from build123d import *

# Parameters (mm, degrees)
SKETCH1_R                          = 5.1
BOSS_EXTRUDE1_DEPTH                = 70.75
FURO_ROSCADO_DE_M5X0_81_AT_2_COUNT = 2
FURO_ROSCADO_DE_M5X0_81_AT_2_PITCH = 32
M3X0_5_TAPPED_HOLE1_AT_2_COUNT     = 2
M3X0_5_TAPPED_HOLE1_AT_2_PITCH     = 11.313708499
M3X0_5_TAPPED_HOLE1_AT_3_COUNT     = 2
M3X0_5_TAPPED_HOLE1_AT_3_PITCH     = 11.313708499
M3X0_5_TAPPED_HOLE1_AT_4_COUNT     = 2
M3X0_5_TAPPED_HOLE1_AT_4_PITCH     = 16
FURO_ROSCADO_DE_M4X0_71_AT_2_COUNT = 2
FURO_ROSCADO_DE_M4X0_71_AT_2_PITCH = 42
PADR_O_LINEAR1_COUNT               = 2
PADR_O_LINEAR1_PITCH               = 180
SKETCH5_W                          = 100
SKETCH5_H                          = 30
BOSS_EXTRUDE2_DEPTH                = 141.5
LPATTERN1_COUNT                    = 2
LPATTERN1_PITCH                    = 140


with BuildPart() as part:
    # Sketch1 → Boss-Extrude1 (new, symmetric)
    with BuildSketch(Plane.XY):
        with BuildLine():
            Line((-140, 0), (-140, 26))
            Line((-140, 26), (140, 26))
            Line((140, 26), (140, 0))
            Line((140, 0), (101.674330816, 0))
            ThreePointArc((101.674330816, 0), (90, 7.7), (78.325669184, 0))
            Line((78.325669184, 0), (-78.325669184, 0))
            ThreePointArc((-78.325669184, 0), (-90, 7.7), (-101.674330816, 0))
            Line((-101.674330816, 0), (-140, 0))
        make_face()
        with Locations((0, 15)):
            Circle(SKETCH1_R, mode=Mode.SUBTRACT)
    extrude(amount=BOSS_EXTRUDE1_DEPTH, both=True)

    # Esboço3 → Furo roscado de M5x0.81 (revolve, cut)
    with BuildSketch(Plane(origin=(110, 26, -50), x_dir=(0, 0, 1), z_dir=(1, 0, 0))):
        Polygon((0, 0), (0, 15.2618073), (2.1, 14), (2.1, 0.425), (2.525, 0), align=None)
    furo_roscado_de_m5x0_81 = revolve(axis=Axis((110, 32.35, -50), (0, -1, 0)), mode=Mode.SUBTRACT)

    # Furo roscado de M5x0.81 at 2: Furo roscado de M5x0.81 ×2
    with Locations(*[(0, 0, i * FURO_ROSCADO_DE_M5X0_81_AT_2_PITCH) for i in range(1, FURO_ROSCADO_DE_M5X0_81_AT_2_COUNT)]):
        add(furo_roscado_de_m5x0_81, mode=Mode.SUBTRACT)

    # Sketch4 → M3x0.5 Tapped Hole1 (revolve, cut)
    with BuildSketch(Plane(origin=(-5.656854249, 20.656854249, 70.75), x_dir=(0, -1, 0), z_dir=(1, 0, 0))):
        Polygon((0, 0), (0, 13.251075774), (1.25, 12.5), (1.25, 0), align=None)
    m3x0_5_tapped_hole1 = revolve(axis=Axis((-5.656854249, 20.656854249, 77.1), (0, 0, -1)), mode=Mode.SUBTRACT)

    # M3x0.5 Tapped Hole1 at 2: M3x0.5 Tapped Hole1 ×2
    with Locations(*[(i * M3X0_5_TAPPED_HOLE1_AT_2_PITCH, 0, 0) for i in range(1, M3X0_5_TAPPED_HOLE1_AT_2_COUNT)]):
        add(m3x0_5_tapped_hole1, mode=Mode.SUBTRACT)

    # M3x0.5 Tapped Hole1 at 3: M3x0.5 Tapped Hole1 ×2
    with Locations(*[(0, -i * M3X0_5_TAPPED_HOLE1_AT_3_PITCH, 0) for i in range(1, M3X0_5_TAPPED_HOLE1_AT_3_COUNT)]):
        add(m3x0_5_tapped_hole1, mode=Mode.SUBTRACT)

    # M3x0.5 Tapped Hole1 at 4: M3x0.5 Tapped Hole1 ×2
    with Locations(*[Vector(0.7071067811865596, -0.7071067811865357, 0) * (i * M3X0_5_TAPPED_HOLE1_AT_4_PITCH) for i in range(1, M3X0_5_TAPPED_HOLE1_AT_4_COUNT)]):
        add(m3x0_5_tapped_hole1, mode=Mode.SUBTRACT)

    # Mirror2: M3x0.5 Tapped Hole1 across plane
    add(m3x0_5_tapped_hole1.mirror(Plane.XY), mode=Mode.SUBTRACT)

    # Mirror2 copy 1 sketch → Mirror2 copy 1 (revolve, cut)
    with BuildSketch(Plane(origin=(5.656854249, 20.656854249, -70.75), x_dir=(0, -1, 0), z_dir=(1, 0, 0))):
        Polygon((0, 0), (0, -13.251075774), (1.25, -12.5), (1.25, 0), align=None)
    revolve(axis=Axis((5.656854249, 20.656854249, -77.1), (0, 0, -1)), mode=Mode.SUBTRACT)

    # Mirror2 copy 2 sketch → Mirror2 copy 2 (revolve, cut)
    with BuildSketch(Plane(origin=(-5.656854249, 9.343145751, -70.75), x_dir=(0, -1, 0), z_dir=(1, 0, 0))):
        Polygon((0, 0), (0, -13.251075774), (1.25, -12.5), (1.25, 0), align=None)
    revolve(axis=Axis((-5.656854249, 9.343145751, -77.1), (0, 0, -1)), mode=Mode.SUBTRACT)

    # Mirror2 copy 3 sketch → Mirror2 copy 3 (revolve, cut)
    with BuildSketch(Plane(origin=(5.656854249, 9.343145751, -70.75), x_dir=(0, -1, 0), z_dir=(1, 0, 0))):
        Polygon((0, 0), (0, -13.251075774), (1.25, -12.5), (1.25, 0), align=None)
    revolve(axis=Axis((5.656854249, 9.343145751, -77.1), (0, 0, -1)), mode=Mode.SUBTRACT)

    # Esboço7 → Furo roscado de M4x0.71 (revolve, cut)
    with BuildSketch(Plane(origin=(-55, 26, -21), x_dir=(0, 0, 1), z_dir=(1, 0, 0))):
        Polygon((0, 0), (0, 12.491420021), (1.65, 11.5), (1.65, 0.375), (2.025, 0), align=None)
    furo_roscado_de_m4x0_71 = revolve(axis=Axis((-55, 32.35, -21), (0, -1, 0)), mode=Mode.SUBTRACT)

    # Furo roscado de M4x0.71 at 2: Furo roscado de M4x0.71 ×2
    with Locations(*[(0, 0, i * FURO_ROSCADO_DE_M4X0_71_AT_2_PITCH) for i in range(1, FURO_ROSCADO_DE_M4X0_71_AT_2_COUNT)]):
        add(furo_roscado_de_m4x0_71, mode=Mode.SUBTRACT)

    # Padrão linear1: Furo roscado de M4x0.71 ×2
    with Locations(*[(i * PADR_O_LINEAR1_PITCH, 0, 0) for i in range(1, PADR_O_LINEAR1_COUNT)]):
        add(furo_roscado_de_m4x0_71, mode=Mode.SUBTRACT)

    # Padrão linear1 copy 1 sketch → Padrão linear1 copy 1 (revolve, cut)
    with BuildSketch(Plane(origin=(125, 26, 21), x_dir=(0, 0, 1), z_dir=(1, 0, 0))):
        Polygon((0, 0), (0, 12.491420021), (1.65, 11.5), (1.65, 0.375), (2.025, 0), align=None)
    revolve(axis=Axis((125, 32.35, 21), (0, -1, 0)), mode=Mode.SUBTRACT)

    # Sketch5 → Boss-Extrude2 (add)
    with BuildSketch(Plane.XY.offset(70.75)):
        with Locations((0, -15)):
            Rectangle(SKETCH5_W, SKETCH5_H)
    extrude(amount=-BOSS_EXTRUDE2_DEPTH)

    # LPattern1: Furo roscado de M5x0.81 ×2
    with Locations(*[(-i * LPATTERN1_PITCH, 0, 0) for i in range(1, LPATTERN1_COUNT)]):
        add(furo_roscado_de_m5x0_81, mode=Mode.SUBTRACT)

    # LPattern1 copy 1 sketch → LPattern1 copy 1 (revolve, cut)
    with BuildSketch(Plane(origin=(-30, 26, -18), x_dir=(0, 0, 1), z_dir=(1, 0, 0))):
        Polygon((0, 0), (0, 15.2618073), (2.1, 14), (2.1, 0.425), (2.525, 0), align=None)
    revolve(axis=Axis((-30, 32.35, -18), (0, -1, 0)), mode=Mode.SUBTRACT)

    # Mirror3: Furo roscado de M5x0.81 across plane
    add(furo_roscado_de_m5x0_81.mirror(Plane.XY), mode=Mode.SUBTRACT)

    # Mirror3 copy 1 sketch → Mirror3 copy 1 (revolve, cut)
    with BuildSketch(Plane(origin=(110, 26, 18), x_dir=(0, 0, -1), z_dir=(1, 0, 0))):
        Polygon((0, 0), (0, -15.2618073), (2.1, -14), (2.1, -0.425), (2.525, 0), align=None)
    revolve(axis=Axis((110, 32.35, 18), (0, 1, 0)), mode=Mode.SUBTRACT)

    # Mirror3 copy 2 sketch → Mirror3 copy 2 (revolve, cut)
    with BuildSketch(Plane(origin=(-30, 26, 50), x_dir=(0, 0, -1), z_dir=(1, 0, 0))):
        Polygon((0, 0), (0, -15.2618073), (2.1, -14), (2.1, -0.425), (2.525, 0), align=None)
    revolve(axis=Axis((-30, 32.35, 50), (0, 1, 0)), mode=Mode.SUBTRACT)

    # Mirror3 copy 3 sketch → Mirror3 copy 3 (revolve, cut)
    with BuildSketch(Plane(origin=(-30, 26, 18), x_dir=(0, 0, -1), z_dir=(1, 0, 0))):
        Polygon((0, 0), (0, -15.2618073), (2.1, -14), (2.1, -0.425), (2.525, 0), align=None)
    revolve(axis=Axis((-30, 32.35, 18), (0, 1, 0)), mode=Mode.SUBTRACT)


solid = part.part
Geometry check sheet. Reference: the model listing, model coordinates, mm. A direction names the side the tool comes from. Give positions to 0.01 mm unless a question says otherwise; leave off trailing zeros. Order: outer loops, then holes, each group sorted by start corner. A loop starts at its lowest first (then second) coordinate and runs counter-clockwise, first axis right, second up. Notation, with made-up numbers: (-38.5, 7.5) - (-22.5, 7.5) arc R18 ccw to (-22.5, 21.5) - close; hole circle Ø11 at (5, 67). An arc over 180 degrees is marked (long way). Use one line per item in the form item = value.
1) Sectioned sample at C-C (x = -70.5). Record the boundary of the cut face in (y, z), and give its area (3 significant figures).
Working result:
outline = (0, -70.75) - (26, -70.75) - (26, 70.75) - (0, 70.75) - close
area = 3,680 mm^2
2) Material ranges on probe 1 along Z at (x, y) = (-30, 17.5); probe 2 along X at (y, z) = (18.25, 18); probe 3 along X at (y, z) = (12, -17), recorded low to high. Write a range as from..to.
Working result:
probe_1 = -70.75..-52.1, -47.9..-20.1, -15.9..15.9, 20.1..47.9, 52.1..70.75
probe_2 = -140..-32.1, -27.9..-3.93, 3.93..107.9, 112.1..140
probe_3 = -140..-31.85, -28.15..-4.12, 4.12..108.15, 111.85..140
3) Access from +Z, -Z, +X, -X, +Y, -Y to the whole of each face (thin tool, end or side, straight path). Record for faces 1 (the face through (64, 0, 1)), 2 (the face through (-2, 26, 1)), 3 (the face through (-64, 0, 1)).
Working result:
face_1 = +Z, -Z, +X, -Y
face_2 = +Z, -Z, +X, -X, +Y
face_3 = +Z, -Z, -X, -Y
4) Sectioned sample at B-B (y = -10). Record the boundary of the cut face in (x, z), and give its area (4 significant figures).
Working result:
outline = (-50, -70.75) - (50, -70.75) - (50, 70.75) - (-50, 70.75) - close
area = 14,150 mm^2
5) Sectioned sample at A-A (x = 0). Record the boundary of the cut face in (y, z).
Working result:
outline = (-30, -70.75) - (9.9, -70.75) - (9.9, 70.75) - (-30, 70.75) - close; (20.1, -70.75) - (26, -70.75) - (26, 70.75) - (20.1, 70.75) - close
6) Depth check by flat-ended pin: pin 1 Ø1.5 at (x, y) = (-5.66, 9.34) entering from -Z; pin 2 Ø4.5 at (x, z) = (-55, -21) entering from -Y; pin 3 Ø4 at (x, y) = (-5.66, 9.34) entering from -Z; pin 4 Ø2.5 at (x, z) = (110, -18) entering from +Y. Enter the tip coordinate at first touch or a pass-through.
Working result:
pin_1 = -57.95
pin_2 = 0
pin_3 = -70.75
pin_4 = 11.49
7) Draft check along X on faces 4 (the face through (2, 5, -70.75)), 5 (the face through (-140, 13, 1)), 6 (the face through (90.2, 7.7, 1)). Enter one of: released by +X, released by -X, zero draft, split by the parting line, or undercut.
Working result:
face_4 = zero draft
face_5 = released by -X
face_6 = undercut
